The listing builds one solid part. Answer for the finished solid, in the listing's coordinates (mm). Coordinates: 2 decimals unless noted, no trailing zeros. Order: outer loops, then holes, each group sorted by start corner. A loop starts at its lowest first (then second) coordinate and runs counter-clockwise, first axis right, second up. Notation, with made-up numbers: (-27.75, 0.25) - (7.25, 0.25) arc R15 cw to (7.25, 6.25) - close; hole circle Ø2 at (52.25, 23.25). An arc over 180 degrees is marked (long way). Use one line per item in the form item = value. Start each with the question number.
Item 1: Section A-A, the plane z = 0.5 is taken. Write down the section's boundary in (x, y), and give its area (3 significant figures).
Item 2: Consider line 1 along X through (y, z) = (1, 2.5); line 2 along X through (y, z) = (-0.5, -3.75); line 3 along Y through (x, z) = (44.5, 0.5). Determine where each line is inside the solid, lowest interval first. Write a range as [from, to].
Item 3: Section B-B, the plane y = 3 is taken. Write down the section's boundary in (x, z), and give its area (3 significant figures).
Item 4: Each of these flat-tipped pins is pushed along its axis until it touches: pin 1 Ø1.5 at (y, z) = (4.5, -2.5) entering from -X; pin 2 Ø6 at (y, z) = (-6, 0.5) entering from -X. Where does it stop, or does it pass through?
Autodesk Inventor part; units mm, degrees
ref_plane "Work Plane1" through (0, 0, -7) normal (0, 0, 1) x (1, 0, 0)
ref_plane "Work Plane2" through (0, 0, 4) normal (0, 0, 1) x (1, 0, 0)
ref_plane "Work Plane3" through (50, 0, 4) normal (1, 0, 0) x (0, 1, 0)
sketch "草图1" plane through (0, 0, 0) normal (0, 0, 1) x (1, 0, 0)
  line L0 (9, 9) -> (41, 9)
  line L1 (41, -9) -> (9, -9)
  arc A0 (9, 9) -> (9, -9) centre (9, 0) ccw
  line L2 (0, 9.4) -> (0, -7.4)
  line L3 (-5, 0) -> (30, 0)
  arc A1 (41, -9) -> (41, 9) centre (41, 0) ccw
  line L4 (50, 0) -> (50, 7) construction
  dimension "d0" = 9
  dimension "d8" = 9
  dimension "d9" = 50
ref_plane "Work Plane1" through (0, 0, -7) normal (0, 0, 1) x (1, 0, 0)
ref_plane "Work Plane2" through (0, 0, 4) normal (0, 0, 1) x (1, 0, 0)
extrude "轴承体1" add sketch "草图1" against normal up to surface (11 mm away) from surface at 4
ref_plane "Work Plane3" through (50, 0, 4) normal (1, 0, 0) x (0, 1, 0)
equation "\"d0\" = 0.5 * PB"
equation "\"d8\" = 0.5 * PB"
equation "\"d9\" = NLG"
equation "\"d1\" = -PNT"
equation "\"d2\" = PH - PNT"
equation "\"NLG\" = 50"
equation "\"PB\" = 18"
equation "\"PNT\" = 7"
equation "\"PH\" = 11"
equation "\"RR\" = 0.001"
equation "\"WDMIN\" = 58"
equation "\"PHH\" = 0"
equation "\"WDMAX\" = 65"
equation "\"PUEB\" = 4.4"
properties part number "DIN 6885 - A 18 x 11 x 50" material "钢，软"
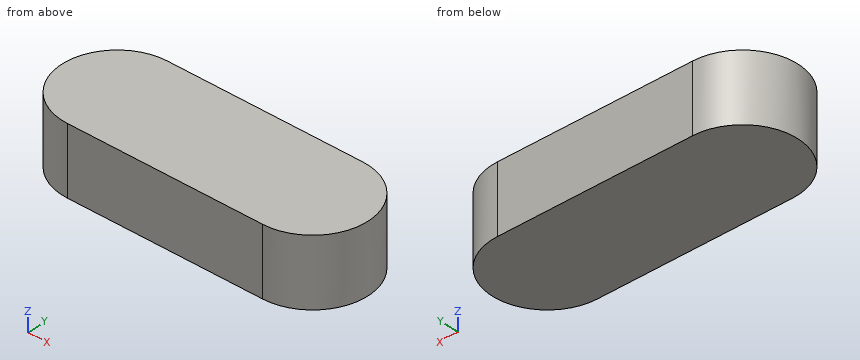
Response:
q1.outline = (9, -9) - (41, -9) arc R9 ccw to (41, 9) - (9, 9) arc R9 ccw to start
q1.area = 830 mm2
q2.line_1 = [0.06, 49.94]
q2.line_2 = [0.01, 49.99]
q2.line_3 = [-8.29, 8.29]
q3.outline = (0.51, -7) - (49.49, -7) - (49.49, 4) - (0.51, 4) - close
q3.area = 539 mm2
q4.pin_1 = 0.82
q4.pin_2 = 0.51
